```python
from build123d import *

# Parameters (mm, degrees)
BOSS_EXTRUDE1_DEPTH = 12.7
SKETCH4_R           = 2.54
CUT_EXTRUDE3_DEPTH  = 43.063657711
CUT_EXTRUDE6_DEPTH  = 5.08


with BuildPart() as part:
    # Sketch3 → Boss-Extrude1 (new body)
    with BuildSketch(Plane(origin=(0, 0, 0), x_dir=(1, 0, 0), z_dir=(0, 1, 0))):
        with BuildLine():
            Line((-31.75, 7.62), (31.75, 7.62))
            ThreePointArc((31.75, 7.62), (39.37, 0), (31.75, -7.62))
            Line((31.75, -7.62), (-31.75, -7.62))
            ThreePointArc((-31.75, -7.62), (-39.37, 0), (-31.75, 7.62))
        make_face()
    extrude(amount=BOSS_EXTRUDE1_DEPTH)

    # Sketch4 → Cut-Extrude3 (cut, through all)
    with BuildSketch(Plane(origin=(0, 12.7, 0), x_dir=(1, 0, 0), z_dir=(0, 1, 0))):
        with Locations(Location((-31.75, 0, 0), (0, 0, 270))):
            Circle(SKETCH4_R)
    extrude(amount=-CUT_EXTRUDE3_DEPTH, mode=Mode.SUBTRACT)

    # Sketch9 → Cut-Extrude6 (cut)
    with BuildSketch(Plane(origin=(0, 12.7, 0), x_dir=(-1, 0, 0), z_dir=(0, 1, 0))):
        with BuildLine():
            Line((1.467889357, -2.490486745), (-10.397234737, -3.528550595))
            ThreePointArc((-10.397234737, -3.528550595), (-15.25, -6), (-20.102765263, -3.528550595))
            Line((-20.102765263, -3.528550595), (-31.967889357, -2.490486745))
            ThreePointArc((-31.967889357, -2.490486745), (-34.25, 0), (-31.967889357, 2.490486745))
            Line((-31.967889357, 2.490486745), (-20.102765263, 3.528550595))
            ThreePointArc((-20.102765263, 3.528550595), (-15.25, 6), (-10.397234737, 3.528550595))
            Line((-10.397234737, 3.528550595), (1.467889357, 2.490486745))
            ThreePointArc((1.467889357, 2.490486745), (3.75, 0), (1.467889357, -2.490486745))
        make_face()
    extrude(amount=-CUT_EXTRUDE6_DEPTH, mode=Mode.SUBTRACT)


solid = part.part
```
Check sheet for the modelled part. Datum: model origin and axes. Units: mm. A direction names the side the tool comes from. Give positions to 0.01 mm unless a question says otherwise; leave off trailing zeros. Write each loop counter-clockwise with the first axis right and the second up, starting at its lowest first coordinate (ties: lowest second). Pieces come first, ordered by that corner, then holes.
Item 1: Cross-section at B-B (y = 5). Enter the section's corners in (x, z), and give its area (3 significant figures).
Item 2: Cross-section at C-C (x = 9). Enter the section's corners in (y, z).
Item 3: Cross-section at A-A (z = 0). Enter the section's corners in (x, y), and give its area (3 significant figures).
Item 4: Scan lines: L1, parallel to X at y = 9.75, z = 0; L2, parallel to X at y = 4.75, z = 0; L3, parallel to Y at x = 12.5, z = 3.5. Record each from-to range of solid material in increasing order.
Item 5: Cross-section at D-D (x = 31). Enter the section's corners in (y, z).
Item 6: Access from +Z, -Z, +X, -X, +Y, -Y to the whole of each face (thin tool, end or side, straight path). Record for faces 5 (the face through (34.25, 10.2, -0.05)), 6 (the face through (1, 0, 0)).
Item 7: Draft check along Z on faces 1 (the face through (39.37, 6.26, -0.17)), 2 (the face through (4.382, 10.196, -3.002)), 3 (the face through (-8, 12.7, 0)), 4 (the face through (4.548, 10.196, 3.017)). Enter one of: released by +Z, released by -Z, zero draft, split by the parting line, or undercut.
Item 8: Gauge pin test, flat ends, axial feed: pin 1 (4 mm diameter, centred on y = 11, z = -5.5, fed in from -X); pin 2 (4 mm diameter, centred on y = 5.5, z = 4, fed in from +X). Record the tip position at first contact, or that the pin passes through.
Report:
1. outline: (-31.75, -7.62) - (31.75, -7.62) arc R7.62 ccw to (31.75, 7.62) - (-31.75, 7.62) arc R7.62 ccw to start; hole circle Ø5.08 at (-31.75, 0)
1. area: 1,130 mm2
2. outline: (0, -7.62) - (12.7, -7.62) - (12.7, -3.41) - (7.62, -3.41) - (7.62, 3.41) - (12.7, 3.41) - (12.7, 7.62) - (0, 7.62) - close
3. outline: (-39.37, 0) - (-34.29, 0) - (-34.29, 12.7) - (-39.37, 12.7) - close; (-29.21, 0) - (39.37, 0) - (39.37, 12.7) - (34.25, 12.7) - (34.25, 7.62) - (-3.75, 7.62) - (-3.75, 12.7) - (-29.21, 12.7) - close
3. area: 742 mm2
4. L1: x = -39.37 to -34.29, -29.21 to -3.75, 34.25 to 39.37
4. L2: x = -39.37 to -34.29, -29.21 to 39.37
4. L3: y = 0 to 7.62
5. outline: (0, -7.62) - (12.7, -7.62) - (12.7, -2.58) - (7.62, -2.58) - (7.62, 2.58) - (12.7, 2.58) - (12.7, 7.62) - (0, 7.62) - close
6. face 5: +Y
6. face 6: +Z, -Z, +X, -X, -Y
7. face 1: split by the parting line
7. face 2: undercut
7. face 3: zero draft
7. face 4: undercut
8. pin 1: stops at x = -38.52
8. pin 2: stops at x = 39.1
